Autodesk Inventor part; units mm, degrees
ref_plane "YZ Plane" through (0, 0, 0) normal (1, 0, 0) x (0, 1, 0)
ref_plane "XZ Plane" through (0, 0, 0) normal (0, 1, 0) x (-1, 0, 0)
ref_plane "XY Plane" through (0, 0, 0) normal (0, 0, 1) x (1, 0, 0)
sketch "Sketch1" plane through (0, 0, 0) normal (0, 0, 1) x (1, 0, 0)
  line L0 (-6.8145, -6.5958) -> (-4.5145, -6.5958)
  line L1 (-4.5145, -6.5958) -> (-3.8195, -7.1258)
  line L2 (-3.8195, -7.1258) -> (-0.9895, -7.1258)
  line L3 (-0.9895, -7.1258) -> (-0.2945, -6.5958)
  line L4 (-0.2945, -6.5958) -> (4.8955, -6.5958)
  line L5 (4.8955, -6.5958) -> (5.5905, -7.1258)
  line L6 (5.5905, -7.1258) -> (8.4205, -7.1258)
  line L7 (8.4205, -7.1258) -> (9.1155, -6.5958)
  line L8 (9.1155, -6.5958) -> (11.5455, -6.5958)
  line L9 (12.2455, -5.8958) -> (12.2455, 2.1742)
  line L10 (11.5455, 2.8742) -> (2.5355, 2.8742)
  line L11 (-7.5145, 2.8542) -> (-7.5145, -5.8958)
  line L12 (-2.4045, -0.6574) -> (-2.4045, -6.9746)
  line L13 (7.0055, -0.6574) -> (7.0055, -6.9746)
  line L14 (-8.0311, -4.1558) -> (13.5632, -4.1558)
  circle A0 centre (-2.4045, -4.1558) radius 1.25
  circle A1 centre (7.0055, -4.1558) radius 1.25
  line L15 (1.9155, 3.5542) -> (2.5355, 2.8742)
  line L16 (-4.4145, 3.5542) -> (-4.4145, 4.2242)
  line L17 (-3.9145, 4.7242) -> (45.5855, 4.7242)
  line L18 (45.5855, 4.7242) -> (45.5855, 4.2442)
  line L19 (45.5855, 4.2442) -> (-3.4345, 4.2442)
  line L20 (-3.9345, 3.7442) -> (-3.9345, 3.5542)
  line L21 (-6.8145, 3.5542) -> (-4.4145, 3.5542)
  line L22 (-3.9345, 3.5542) -> (1.9155, 3.5542)
  arc A2 (-6.8145, 3.5542) -> (-7.5145, 2.8542) centre (-6.8145, 2.8542) ccw
  arc A3 (-7.5145, -5.8958) -> (-6.8145, -6.5958) centre (-6.8145, -5.8958) ccw
  arc A4 (11.5455, -6.5958) -> (12.2455, -5.8958) centre (11.5455, -5.8958) ccw
  arc A5 (12.2455, 2.1742) -> (11.5455, 2.8742) centre (11.5455, 2.1742) ccw
  arc A6 (-3.9145, 4.7242) -> (-4.4145, 4.2242) centre (-3.9145, 4.2242) ccw
  arc A7 (-3.4345, 4.2442) -> (-3.9345, 3.7442) centre (-3.4345, 3.7442) ccw
  point P0 (-7.5145, -6.5958)
  point P1 (12.2455, 2.8742)
  point P2 (-7.5145, 3.5542)
  point P3 (-4.4145, 4.7242)
  dimension "d21" = 2.5
  dimension "d22" = 2.5
  dimension "d23" = 2.97
  dimension "d24" = 0.53
  dimension "d25" = 2.83
  dimension "d26" = 3
  dimension "d27" = 5.11
  dimension "d28" = 9.41
  dimension "d29" = 19.76
  dimension "d31" = 9.47
  dimension "d32" = 9.71
  dimension "d33" = 9.43
  dimension "d40" = 10.15
  dimension "d41" = 3.1
  dimension "d42" = 0.48
  dimension "d43" = 0.48
  dimension "d44" = 1.17
  dimension "d45" = 50
  dimension "d46" = 0.7
  dimension "d47" = 0.5
extrude "Extrusion1" add sketch "Sketch1" along normal blind 6.26 contours A3 L11 L14 A0 A1 L9 A4 L8 L7 L6 L5 L4 L3 L2 L1 L0 | L11 A2 L21 L16 A6 L17 L18 L19 A7 L20 L22 L15 L10 A5 L9 L14 A1 A0
sketch "Sketch2" plane through (0, 0, 6.26) normal (0, 0, 1) x (1, 0, 0)
  line L0 (-3.9345, 3.5542) -> (-3.9345, 3.7442)
  arc A0 (-3.4345, 4.2442) -> (-3.9345, 3.7442) centre (-3.4345, 3.7442) ccw
  line L1 (-3.4345, 4.2442) -> (45.5855, 4.2442)
  line L2 (45.5855, 4.2442) -> (45.5855, 4.7242)
  line L3 (45.5855, 4.7242) -> (-3.9145, 4.7242)
  arc A1 (-3.9145, 4.7242) -> (-4.4145, 4.2242) centre (-3.9145, 4.2242) ccw
  line L4 (-4.4145, 4.2242) -> (-4.4145, 3.5542)
  line L5 (-7.5145, 2.8542) -> (-7.5145, -5.8958)
  line L6 (-4.4145, 3.5542) -> (-3.9345, 3.5542)
  point P0 (0, 0)
extrude "Extrusion2" cut sketch "Sketch2" against normal blind 0.96
sketch "Sketch3" plane through (0, 0, 0) normal (0, 0, -1) x (-1, 0, 0)
  line L0 (4.4145, 3.5542) -> (4.4145, 4.2242)
  arc A0 (4.4145, 4.2242) -> (3.9145, 4.7242) centre (3.9145, 4.2242) ccw
  line L1 (3.9145, 4.7242) -> (-45.5855, 4.7242)
  line L2 (-45.5855, 4.7242) -> (-45.5855, 4.2442)
  line L3 (-45.5855, 4.2442) -> (3.4345, 4.2442)
  arc A1 (3.9345, 3.7442) -> (3.4345, 4.2442) centre (3.4345, 3.7442) ccw
  line L4 (3.9345, 3.7442) -> (3.9345, 3.5542)
  line L5 (0.9895, -7.1258) -> (3.8195, -7.1258)
  line L6 (3.9345, 3.5542) -> (4.4145, 3.5542)
  point P0 (0, 0)
extrude "Extrusion3" cut sketch "Sketch3" against normal blind 1.22
sketch "Sketch4" plane through (-0.2945, -6.5958, 0) normal (0, -1, 0) x (1, 0, 0)
  line L0 (3.09, 4.71) -> (3.67, 4.71)
  line L1 (3.67, 4.71) -> (3.67, 1.43)
  line L2 (3.67, 1.43) -> (3.09, 1.43)
  line L3 (3.09, 1.43) -> (3.09, 4.71)
  line L4 (-5.74, 4.71) -> (-5.16, 4.71)
  line L5 (-5.16, 4.71) -> (-5.16, 1.43)
  line L6 (-5.16, 1.43) -> (-5.74, 1.43)
  line L7 (-5.74, 1.43) -> (-5.74, 4.71)
  line L8 (10.38, 4.71) -> (10.96, 4.71)
  line L9 (10.96, 4.71) -> (10.96, 1.43)
  line L10 (10.96, 1.43) -> (10.38, 1.43)
  line L11 (10.38, 1.43) -> (10.38, 4.71)
  line L12 (-6.52, 6.26) -> (-4.22, 6.26)
  line L13 (-7.22, 0) -> (-7.22, 6.26)
  point P0 (0.2945, 0)
  dimension "d52" = 3.28
  dimension "d54" = 0.58
  dimension "d55" = 1.55
  dimension "d56" = 1.48
  dimension "d57" = 9.41
  dimension "d58" = 7.87
extrude "Extrusion4" add sketch "Sketch4" along normal blind 4.11
sketch "Sketch5" plane through (-6.0345, -10.7058, 1.43) normal (-1, 0, 0) x (0, 0, 1)
  line L0 (0, 4.11) -> (0, 0)
  line L1 (3.28, 0) -> (0, 0)
  line L2 (3.28, 4.11) -> (3.28, 0)
  circle A0 centre (1.64, 1.86) radius 0.77
  line L3 (0, 0.5657) -> (0.5657, 0)
  line L4 (0, 0.5657) -> (0.8, 0.5657) construction
  line L5 (2.7143, 0) -> (3.28, 0.5657)
  point P0 (-1.43, 10.7058)
  dimension "d61" = 1.54
  dimension "d62" = 1.86
  dimension "d63" = 3.28
  dimension "d64" = 1.64
  dimension "d65" = 45
  dimension "d66" = 0.8
extrude "Extrusion5" cut sketch "Sketch5" against normal through all
equation "\"d22\" = d21"
equation "\"d43\" = d42"
equation "\"d64\" = 0.5 * d63"
equation "\"d7\" = d6"
properties part number "switch" material "Acetal Resin, Black"
Work out the finished part from the listing and answer in its coordinate system (mm). A direction names the side the tool comes from. Coordinates: 2 decimals unless noted, no trailing zeros. Write each loop counter-clockwise with the first axis right and the second up, starting at its lowest first coordinate (ties: lowest second). Pieces come first, ordered by that corner, then holes.
1. The part is cut by section A-A, the plane z = 3.07. State how many separate pieces and enclosed holes the cut face has, and give its area (3 significant figures).
Results list:
separate pieces: 4
enclosed holes: 2
area: 216 mm2
2. Flat-ended cylindrical pins translate along their axes: pin 1 (1.6 mm diameter, centred on y = -8, z = 2.5, fed in from +X); pin 2 (1.6 mm diameter, centred on y = -8, z = 2.5, fed in from -X); pin 3 (0.8 mm diameter, centred on x = -2.5, z = 3.5, fed in from -Y). Find the tip coordinate at first contact, or state that the pin passes through.
Results list:
pin 1: stops at x = 10.67
pin 2: stops at x = -6.03
pin 3: stops at y = -7.13
3. For a pull along Y with two mould halves and no side action, classify faces 1 (the flat face through (7, -7.126, 3)), 2 (the cylindrical face through (-2.675, -2.936, 3.086)), 3 (the flat face through (10.666, -9, 4)) as +Y half, -Y half, draft (parallel to the pull), parting line (faces both ways), or undercut.
Results list:
face 1: -Y half
face 2: undercut
face 3: draft
4. For faces 4 (the flat face through (12.246, -2, 3)), 5 (the flat face through (20.2, 4.4, 5.3)), 6 (the flat face through (-6.034, -9, 2)), 7 (the flat face through (20.9, 4.4, 1.22)), 8 (the flat face through (-5.454, -9, 4)), determine the directions among +Z, -Z, +X, -X, +Y, -Y from which every point of the face is accessible in a straight line to the end or side of a thin tool.
Results list:
face 4: +Z, -Z, +X, -Y
face 5: +Z, +X, -X, +Y
face 6: +Z, -Z, -X, -Y
face 7: -Z, +X, -X, +Y
face 8: +Z, -Z, -Y
5. Consider line 1 along Y through (x, z) = (3.25, 3.07); line 2 along X through (y, z) = (-9, 4.5); line 3 along Y through (x, z) = (-5.7, 3.07). Determine where each line is inside the solid, lowest interval first.
Results list:
line 1: y = -10.71 to -9.62, -8.08 to 2.87, 4.24 to 4.72
line 2: x = -6.03 to -5.45, 2.8 to 3.38, 10.09 to 10.67
line 3: y = -10.71 to -9.62, -8.08 to 3.55
6. The part is cut by section B-B, the plane y = -3.5. Write down the section's boundary in (x, z).
Results list:
outline: (-7.51, 0) - (-3.47, 0) - (-3.47, 6.26) - (-7.51, 6.26) - close; (-1.34, 0) - (5.94, 0) - (5.94, 6.26) - (-1.34, 6.26) - close; (8.07, 0) - (12.25, 0) - (12.25, 6.26) - (8.07, 6.26) - close
7. The part is cut by section D-D, the plane y = -1.5. Write down the section's boundary in (x, z), and give its area (3 significant figures).
Results list:
outline: (-7.51, 0) - (12.25, 0) - (12.25, 6.26) - (-7.51, 6.26) - close
area: 124 mm2
8. The part is cut by section C-C, the plane x = 14.5. Write down the section's boundary in (y, z), and give its area (3 significant figures).
Results list:
outline: (4.24, 1.22) - (4.72, 1.22) - (4.72, 5.3) - (4.24, 5.3) - close
area: 1.96 mm2
